from build123d import *

# Parameters (mm, degrees)
SKETCH1_W           = 75.2
SKETCH1_H           = 261
BOSS_EXTRUDE1_DEPTH = 3
SKETCH2_W           = 5
SKETCH2_H           = 67
CUT_EXTRUDE1_DEPTH  = 136.841856583
SKETCH3_W           = 2
SKETCH3_H           = 20
CUT_EXTRUDE2_DEPTH  = 136.841856583


with BuildPart() as part:
    # Sketch1 → Boss-Extrude1 (new body)
    with BuildSketch(Plane(origin=(0, 0, 0), x_dir=(1, 0, 0), z_dir=(0, 1, 0))):
        Rectangle(SKETCH1_W, SKETCH1_H)
    extrude(amount=BOSS_EXTRUDE1_DEPTH)

    # Sketch2 → Cut-Extrude1 (cut, through all)
    with BuildSketch(Plane(origin=(0, 3, 0), x_dir=(1, 0, 0), z_dir=(0, 1, 0))):
        Polygon((-37.6, -130.5), (-15, -130.5), (-15, -125.5), (-32.6, -125.5), (-32.6, -63.5), (-37.6, -63.5), align=None)
        with Locations((-35.1, 0)):
            Rectangle(SKETCH2_W, SKETCH2_H)
        Polygon((-37.6, 130.5), (-15, 130.5), (-15, 125.5), (-32.6, 125.5), (-32.6, 63.5), (-37.6, 63.5), align=None)
    cut_extrude1 = extrude(amount=-CUT_EXTRUDE1_DEPTH, mode=Mode.SUBTRACT)

    # Mirror1: Cut-Extrude1 across plane
    add(cut_extrude1.mirror(Plane(origin=(0, 0, 0), x_dir=(0, 0, 1), z_dir=(1, 0, 0))), mode=Mode.SUBTRACT)

    # Sketch3 → Cut-Extrude2 (cut, through all)
    with BuildSketch(Plane(origin=(0, 3, 0), x_dir=(1, 0, 0), z_dir=(0, 1, 0))):
        with Locations((31.6, 108.75)):
            Rectangle(SKETCH3_W, SKETCH3_H)
    extrude(amount=-CUT_EXTRUDE2_DEPTH, mode=Mode.SUBTRACT)


solid = part.part
Geometry check sheet. Reference: the model listing, model coordinates, mm. Round coordinates to 2 decimals unless told otherwise and drop trailing zeros. Loops run counter-clockwise (first coordinate to the right, second up) from the corner with the lowest first, then second, coordinate; pieces in that order, holes last. Notation, with made-up numbers: (89.25, -30) -> (127.25, -30) arc R32 ccw to (127.25, 6) -> close; hole circle Ø4 at (46, 56). An arc over 180 degrees is marked (long way). Answer as a JSON object with one key per item and string values. Group by question number.
Item 1: Cross-section at C-C, the plane x = 18. Record the cut outline in (y, z).
Item 2: Depth check by flat-ended pin: pin 1 Ø1.6 at (x, y) = (31.5, 2) entering from -Z; pin 2 Ø1.5 at (y, z) = (2, 18.5) entering from +X; pin 3 Ø0.9 at (x, y) = (-35, 1) entering from -Z. Enter the tip coordinate at first touch or a pass-through.
Item 3: Cross-section at B-B, the plane z = -69. Record the cut outline in (x, y), plus the area to 3 significant figures.
Item 4: Thickness scan on line 1 along X through (y, z) = (0.35, 74); line 2 along Z through (x, y) = (-18, 1.5); line 3 along X through (y, z) = (0.5, -115). Record the ranges inside material, lowest first.
Determined:
{
 "1": {"outline": "(0, -125.5) -> (3, -125.5) -> (3, 125.5) -> (0, 125.5) -> close"},
 "2": {"pin 1": "stops at z = -125.5", "pin 2": "stops at x = 32.6", "pin 3": "stops at z = -63.5"},
 "3": {"outline": "(-32.6, 0) -> (32.6, 0) -> (32.6, 3) -> (-32.6, 3) -> close", "area": "196 mm²"},
 "4": {"line 1": "x = -32.6 to 32.6", "line 2": "z = -125.5 to 125.5", "line 3": "x = -32.6 to 30.6"}
}
